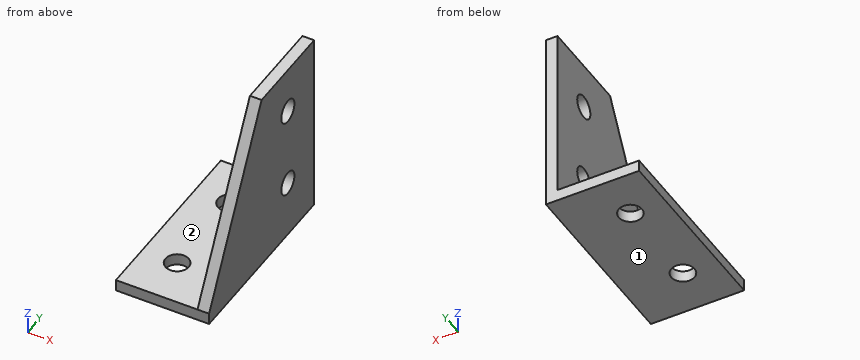
Autodesk Inventor part; units mm, degrees
ref_plane "YZ Plane" through (0, 0, 0) normal (1, 0, 0) x (0, 1, 0)
ref_plane "XZ Plane" through (0, 0, 0) normal (0, 1, 0) x (-1, 0, 0)
ref_plane "XY Plane" through (0, 0, 0) normal (0, 0, 1) x (1, 0, 0)
sketch "Sketch1" plane through (0, 0, 0) normal (1, 0, 0) x (0, 1, 0)
  line L0 (-25.4, 0) -> (-50.8, -47.625)
  line L1 (-50.8, -47.625) -> (-50.8, -50.8)
  line L2 (-50.8, -50.8) -> (0, -50.8)
  line L3 (0, -50.8) -> (0, 0)
  line L4 (0, 0) -> (-25.4, 0)
  circle A0 centre (-12.7, -12.7) radius 3.175
  circle A1 centre (-12.7, -34.925) radius 3.175
  dimension "d1" = 3.175
  dimension "d2" = 50.8
  dimension "d3" = 50.8
  dimension "d4" = 25.4
  dimension "d5" = 6.35
  dimension "d6" = 6.35
  dimension "d7" = 15.875
  dimension "d8" = 12.7
  dimension "d9" = 12.7
  dimension "d10" = 12.7
extrude "Extrusion1" add sketch "Sketch1" along normal blind 3.175
sketch "Sketch2" plane through (0, 0, 0) normal (-1, 0, 0) x (0, 0, 1)
  line L0 (-50.8, -50.8) -> (-50.8, 0)
  line L1 (-50.8, 0) -> (0, 0)
  line L2 (-50.8, -50.8) -> (-47.625, -50.8)
  line L3 (-47.625, -50.8) -> (-47.625, 0)
  line L4 (-47.625, 0) -> (-50.8, 0)
  line L5 (-50.8, 0) -> (-50.8, -50.8)
  dimension "d13" = 3.175
extrude "Extrusion2" add sketch "Sketch2" along normal blind 22.225
sketch "Sketch3" plane through (0, -50.8, -47.625) normal (0, 0, 1) x (1, 0, 0)
  circle A0 centre (-12.7, 12.7) radius 3.175
  circle A1 centre (-12.7, 38.1) radius 3.175
  line L0 (-22.225, 50.8) -> (-22.225, 0)
  line L1 (0, 50.8) -> (-22.225, 50.8)
  line L2 (0, 0) -> (-22.225, 0)
  dimension "d16" = 9.525
  dimension "d17" = 12.7
  dimension "d18" = 9.525
  dimension "d19" = 12.7
  dimension "d20" = 6.35
extrude "Extrusion3" cut sketch "Sketch3" against normal blind 22.225
properties part number "15102898-16-P-0207" material "Aluminum 6061"
For this review, take the finished solid that the model builds, in its own axes (mm). Face numbers are marked on the shaded views. A direction names the side the tool comes from. Give positions to 0.01 mm unless a question says otherwise; leave off trailing zeros. Write each loop counter-clockwise with the first axis right and the second up, starting at its lowest first coordinate (ties: lowest second). Pieces come first, ordered by that corner, then holes. Notation, with made-up numbers: (81.5, 19.5) -> (139.5, 19.5) arc R19 ccw to (139.5, 42.5) -> close; hole circle Ø10 at (22.25, 73.25). An arc over 180 degrees is marked (long way). Use CSV: the item, a comma, the result in double quotes.
Q1. For P1, Ø5, axis at x = 0, z = -5, coming from the -Y side; P2, Ø1.5, axis at y = -14, z = -11.5, coming from the +X side; P3, Ø6.5, axis at x = -5.5, y = -15, coming from the +Z side (3 decimals); P4, Ø8.5, axis at y = -12.7, z = -34.925, coming from the -X side, all flat-tipped, find the tip position at first contact; note any pin that passes through.
Conclusion:
P1,"y = -29.4"
P2,"through"
P3,"z = -47.625"
P4,"x = 0"
Q2. Take a section at C-C, the plane z = -12. Write out the cut boundary in (x, y) (3 decimals).
Conclusion:
outline,"(0, -31.8) -> (3.175, -31.8) -> (3.175, -15.797) -> (0, -15.797) -> close; (0, -9.603) -> (3.175, -9.603) -> (3.175, 0) -> (0, 0) -> close"
Q3. Take a section at B-B, the plane y = -12.7. Write out the cut boundary in (x, z) (3 decimals), then the cut area to 3 significant figures.
Conclusion:
outline,"(-22.225, -50.8) -> (-15.875, -50.8) -> (-15.875, -47.625) -> (-22.225, -47.625) -> close; (-9.525, -50.8) -> (3.175, -50.8) -> (3.175, -38.1) -> (0, -38.1) -> (0, -47.625) -> (-9.525, -47.625) -> close; (0, -31.75) -> (3.175, -31.75) -> (3.175, -15.875) -> (0, -15.875) -> close; (0, -9.525) -> (3.175, -9.525) -> (3.175, 0) -> (0, 0) -> close"
area,"171 mm2"
Q4. Take a section at D-D, the plane y = -4. Write out the cut boundary in (x, z) (3 decimals), then the cut area to 3 significant figures.
Conclusion:
outline,"(-22.225, -50.8) -> (3.175, -50.8) -> (3.175, 0) -> (0, 0) -> (0, -47.625) -> (-22.225, -47.625) -> close"
area,"232 mm2"
Q5. To check wall thickness, follow probe 1 along Z at (x, y) = (1.25, -12.7) (3 decimals); probe 2 along Y at (x, z) = (-12.7, -49.1) (3 decimals); probe 3 along Z at (x, y) = (-17.25, -3) (3 decimals). State the ranges of each line that lie inside material, in increasing order. Write a range as [from, to].
Conclusion:
probe 1,"[-50.8, -38.1], [-31.75, -15.875], [-9.525, 0]"
probe 2,"[-50.8, -41.275], [-34.925, -15.875], [-9.525, 0]"
probe 3,"[-50.8, -47.625]"
Q6. Take a section at A-A, the plane x = -12.7. Write out the cut boundary in (y, z) (3 decimals), then the cut area to 3 significant figures.
Conclusion:
outline,"(-50.8, -50.8) -> (-41.275, -50.8) -> (-41.275, -47.625) -> (-50.8, -47.625) -> close; (-34.925, -50.8) -> (-15.875, -50.8) -> (-15.875, -47.625) -> (-34.925, -47.625) -> close; (-9.525, -50.8) -> (0, -50.8) -> (0, -47.625) -> (-9.525, -47.625) -> close"
area,"121 mm2"
Q7. Tool access review of the marked faces 1 and 2: name each direction out of +Z, -Z, +X, -X, +Y, -Y from which nothing blocks a thin tool from reaching the whole face with its end or side.
Conclusion:
face 1,"-Z, +X, -X, +Y, -Y"
face 2,"+Z, -X, +Y, -Y"
